Autodesk Inventor part; units mm, degrees
ref_plane "Work Plane1" through (-14, 0, 0) normal (1, 0, 0) x (0, 1, 0)
ref_plane "XZ Plane" through (0, 0, 0) normal (0, 1, 0) x (-1, 0, 0)
ref_plane "XY Plane" through (0, 0, 0) normal (0, 0, 1) x (1, 0, 0)
sketch "Sketch1" plane through (0, 0, 0) normal (0, 1, 0) x (-1, 0, 0)
  circle A0 centre (0, 0) radius 16
  circle A1 centre (0, 0) radius 14
  dimension "d0" = 32
  dimension "d1" = 28
extrude "Extrusion1" add sketch "Sketch1" along normal blind 50 contours A1
sketch "Sketch2" plane through (0, 0, 0) normal (0, -1, 0) x (1, 0, 0)
  circle A0 centre (0, 0) radius 16
  dimension "d4" = 32
extrude "Extrusion2" add sketch "Sketch2" against normal blind 11
sketch "Sketch3" plane through (0, 50, 0) normal (0, 1, 0) x (1, 0, 0)
  circle A0 centre (0, 0) radius 16
extrude "Extrusion3" add sketch "Sketch3" against normal blind 11
ref_plane "Work Plane1" through (-14, 0, 0) normal (1, 0, 0) x (0, 1, 0)
sketch "Sketch5" plane through (-14, 0, 0) normal (1, 0, 0) x (0, 1, 0)
  line L0 (39, 14) -> (39, -14) construction
  line L1 (39, 0) -> (11, 0) construction
  line L2 (11, -14) -> (11, 14) construction
  line L3 (39, 0) -> (30, 0) construction
  line L4 (11, 0) -> (20, 0) construction
  circle A0 centre (30, 0) radius 3
  circle A1 centre (20, 0) radius 3
  point P0 (0, 0)
  dimension "d10" = 9
  dimension "d11" = 9
  dimension "d12" = 6
  dimension "d13" = 6
extrude "Extrusion4" cut sketch "Sketch5" along normal blind 8
sketch "Sketch6" plane through (-6, 30, 0) normal (-1, 0, 0) x (0, 0, 1)
  line L0 (-4.6081, 4.2685) -> (5.6465, 4.2685)
  line L1 (5.6465, 4.2685) -> (5.6465, -14.2936)
  line L2 (5.6465, -14.2936) -> (-4.6081, -14.2936)
  line L3 (-4.6081, -14.2936) -> (-4.6081, 4.2685)
  point P0 (0, -30)
extrude "Extrusion5" add sketch "Sketch6" along normal blind 2
sketch "Sketch7" plane through (0, 50, 0) normal (0, 1, 0) x (1, 0, 0)
  circle A0 centre (0, 0) radius 14
  circle A1 centre (0, 0) radius 12
  dimension "d18" = 28
  dimension "d19" = 24
extrude "Extrusion6" cut sketch "Sketch7" against normal blind 3
sketch "Sketch8" plane through (0, 50, 0) normal (0, 1, 0) x (1, 0, 0)
  circle A0 centre (0, 0) radius 12
  line L0 (-12, 0) -> (12, 0)
  arc A1 (12, 0) -> (-12, 0) centre (0, 0) ccw
extrude "Extrusion7" cut sketch "Sketch8" against normal up to surface (3 mm away) contours L0 A0 picked at (2.994, 4.567)
sketch "Sketch9" plane through (0, 0, 0) normal (0, -1, 0) x (1, 0, 0)
  arc A0 (12, 0) -> (-12, 0) centre (0, 0) ccw
  line L0 (12, 0) -> (-12, 0)
  circle A1 centre (0, 0) radius 12
  circle A2 centre (0, 0) radius 14
extrude "Extrusion8" cut sketch "Sketch9" against normal blind 3 contours L0 A0 | A1 L0 | A2
sketch "Sketch10" plane through (0, 3, 0) normal (0, -1, 0) x (1, 0, 0)
  line L0 (0, 0) -> (7, 0) construction
  line L1 (12, 0) -> (-12, 0)
  circle A0 centre (7, 0) radius 4
extrude "Extrusion9" cut sketch "Sketch10" against normal blind 3
properties part number "Middle handle"
Build history of the part. All positions in model axes, mm. A direction names the side the tool comes from. Coordinates: 2 decimals unless noted, no trailing zeros. Order: outer loops, then holes, each group sorted by start corner. A loop starts at its lowest first (then second) coordinate and runs counter-clockwise, first axis right, second up. Notation, with made-up numbers: (25.25, -27.75) - (55.25, -27.75) arc R11 ccw to (55.25, -18.75) - close; hole circle Ø3 at (58, 14.25). An arc over 180 degrees is marked (long way). Write each question's results on one line, items separated by ' | '. Start each with the question number.
Item 1: Band-saw the part on A-A on x = 0. Write the cut outline in (y, z).
Item 2: Flat gauge pins, fed straight in: pin 1 (5 mm diameter, centred on x = -6, z = 3, fed in from -Y); pin 2 (6.5 mm diameter, centred on y = 20.5, z = 0, fed in from -X); pin 3 (5 mm diameter, centred on x = -7.5, y = 14, fed in from +Z). Where does each tip first touch, or does it go through?
Item 3: Mould opens along Z. For faces 6 (the face through (0, 49, 12)), 7 (the face through (-3.47, 5.42, -15.62)), 8 (the face through (0.07, 0, -14.15)) say: released by +Z, released by -Z, zero draft, split by the parting line, or undercut.
Item 4: Band-saw the part on C-C on y = 9. Write the cut outline in (x, z).
Item 5: Wall check: probe 1 along Y at (x, z) = (14.5, 1); probe 2 along Z at (x, y) = (0, 1); probe 3 along Y at (x, z) = (-5, -3.5). Give the ranges that are in metal, low to high. Write a range as [from, to].
Item 6: Band-saw the part on B-B on z = -10.5. Write the cut outline in (x, y), and give its area (3 significant figures).
Item 7: Band-saw the part on D-D on x = -4.5. Write the cut outline in (y, z).
Item 8: Tool access for faces 1 (the face through (-8, 30, 0)), 2 (the face through (-0.07, 39, 14.15)), 3 (the face through (-3.47, 44.58, 15.62)), 4 (the face through (0, 3, 0)), 5 (the face through (12.932, 48.521, 5.362)): list every direction of +Z, -Z, +X, -X, +Y, -Y with a clear straight run to the whole face (end or side of a thin tool).
Numbers:
1) outline: (0, -16) - (11, -16) - (11, -14) - (39, -14) - (39, -16) - (50, -16) - (50, -14) - (47, -14) - (47, 0) - (50, 0) - (50, 12) - (47, 12) - (47, 14) - (50, 14) - (50, 16) - (39, 16) - (39, 14) - (11, 14) - (11, 16) - (0, 16) - (0, 14) - (3, 14) - (3, -14) - (0, -14) - close
2) pin 1: y = 3 | pin 2: x = -14 | pin 3: z = 13.08
3) face 6: undercut | face 7: split by the parting line | face 8: zero draft
4) outline: circle Ø32 at (0, 0)
5) probe 1: [0, 11], [39, 50] | probe 2: [-16, -14], [14, 16] | probe 3: [3, 47]
6) outline: (-12.07, 0) - (-9.26, 0) - (-9.26, 3) - (9.26, 3) - (9.26, 0) - (12.07, 0) - (12.07, 11) - (9.26, 11) - (9.26, 39) - (12.07, 39) - (12.07, 50) - (9.26, 50) - (9.26, 47) - (-9.26, 47) - (-9.26, 50) - (-12.07, 50) - (-12.07, 39) - (-9.26, 39) - (-9.26, 11) - (-12.07, 11) - close | area: 939 mm^2
7) outline: (0, -15.35) - (11, -15.35) - (11, -13.26) - (39, -13.26) - (39, -15.35) - (50, -15.35) - (50, -13.26) - (47, -13.26) - (47, 0) - (50, 0) - (50, 11.12) - (47, 11.12) - (47, 13.26) - (50, 13.26) - (50, 15.35) - (39, 15.35) - (39, 13.26) - (11, 13.26) - (11, 15.35) - (0, 15.35) - (0, 13.26) - (3, 13.26) - (3, -13.26) - (0, -13.26) - close
8) face 1: -X | face 2: none | face 3: +Y, -Y | face 4: -Y | face 5: +Y
